Autodesk Inventor part; units mm, degrees
ref_plane "YZ Plane" through (0, 0, 0) normal (1, 0, 0) x (0, 1, 0)
ref_plane "XZ Plane" through (0, 0, 0) normal (0, 1, 0) x (-1, 0, 0)
ref_plane "XY Plane" through (0, 0, 0) normal (0, 0, 1) x (1, 0, 0)
sketch "Sketch1" plane through (0, 0, 0) normal (0, 1, 0) x (-1, 0, 0)
  line L0 (0, 0) -> (-58, 0)
  line L1 (-58, 0) -> (-58, -20)
  line L2 (-58, -20) -> (0, -20)
  line L3 (0, -20) -> (0, 0)
  line L4 (-58, -10) -> (-54, -10) construction
  arc A0 (-56, -11.8875) -> (-52, -11.8875) centre (-54, -10) ccw
  line L5 (-58, -10) -> (-56, -10) construction
  line L6 (-56, -10) -> (-56, -11.8875)
  line L7 (-56, -10) -> (-56, -8.1125)
  line L8 (-54, -10) -> (-52, -10) construction
  line L9 (-52, -10) -> (-52, -11.8875)
  line L10 (-52, -10) -> (-52, -8.1125)
  arc A1 (-52, -8.1125) -> (-56, -8.1125) centre (-54, -10) ccw
  arc A2 (-58, -12.5617) -> (-58, -7.4383) centre (-54, -10) ccw
  line L11 (0, 0) -> (-10, 0) construction
  line L12 (-10, 0) -> (-10, -5) construction
  line L13 (-10, -20) -> (-10, -15) construction
  circle A3 centre (-10, -5) radius 2.75
  circle A4 centre (-10, -15) radius 2.75
  line L14 (-54, -10) -> (-54, -11.925) construction
  line L15 (-54, -10) -> (-54, -8.075) construction
  circle A5 centre (-54, -8.075) radius 0.3
  circle A6 centre (-54, -11.925) radius 0.3
  line L16 (-58, -10) -> (-31.5, -10) construction
  line L17 (-33.5, -10) -> (-24.5, -10) construction
  line L18 (-35.5, -20) -> (-35.5, 0)
  line L19 (-24.5, -20) -> (-24.5, 0)
  line L20 (-31.5, -10) -> (-33.5, -10) construction
  line L21 (-33.5, -10) -> (-35.5, -10) construction
  line L22 (-24.5, 0) -> (-35.5, 0)
  line L23 (-35.5, 0) -> (-35.5, -20)
  line L24 (-35.5, -20) -> (-24.5, -20)
  line L25 (-24.5, -20) -> (-24.5, 0)
  dimension "d0" = 58
  dimension "d1" = 20
  dimension "d2" = 4
  dimension "d4" = 2
  dimension "d5" = 2
  dimension "d7" = 10
  dimension "d8" = 5
  dimension "d9" = 5
  dimension "d10" = 5.5
  dimension "d11" = 5.5
  dimension "d18" = 1.925
  dimension "d19" = 1.925
  dimension "d20" = 0.6
  dimension "d21" = 0.6
  dimension "d24" = 26.5
  dimension "d25" = 9
  dimension "d32" = 2
  dimension "d33" = 2
extrude "Extrusion2" add sketch "Sketch1" against normal blind 8 contours A2 L1
extrude "Extrusion3" add sketch "Sketch1" along normal blind 5 contours A2 L1
extrude "Extrusion4" add sketch "Sketch1" against normal blind 8 contours L6 L7 A1 L10 L9 A0
extrude "Extrusion8" add sketch "Sketch1" against normal blind 8 contours L3 L2 L19 L0 | L18 L2 L1 A2 L0
extrude "Extrusion9" add sketch "Sketch1" against normal blind 2.5 contours L19 L2 L18 L0
properties part number "LDR_Holder"
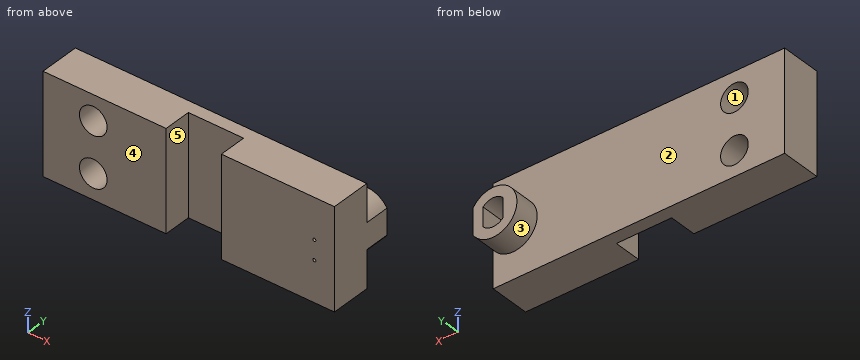
Read the model definition and answer for the solid it produces. Units are mm, in the model's axes. Face numbers are marked on the shaded views. A direction names the side the tool comes from. Give positions to 0.01 mm unless a question says otherwise; leave off trailing zeros. Write each loop counter-clockwise with the first axis right and the second up, starting at its lowest first coordinate (ties: lowest second). Pieces come first, ordered by that corner, then holes. Notation, with made-up numbers: (67, 65) - (103, 65) arc R8 cw to (103, 73) - close; hole circle Ø1 at (-18, 65.25). An arc over 180 degrees is marked (long way). Answer in a Markdown table with one row per item. Add a question column.
Item 1: Section D-D, the plane z = -18.5 is taken. Write down the section's boundary in (x, y).
Item 2: Find the intervals of material crossed by L1, parallel to Z at x = 54, y = -1.75 (3 decimals); L2, parallel to Z at x = 10, y = -6; L3, parallel to X at y = -5.25, z = -1, in increasing order.
Item 3: Flat-ended cylindrical pins translate along their axes: P1, Ø4, axis at y = 3, z = -10, coming from the -X side; P2, Ø4, axis at x = 51, z = -3, coming from the +Y side. Find the tip coordinate at first contact, or state that the pin passes through.
Item 4: Section A-A, the plane x = 10 is taken. Write down the section's boundary in (y, z), and give its area (3 significant figures).
Item 5: A tool of negligible diameter and unlimited length cuts with its end or side. For the marked faces 4 and 5, from which of +Z, -Z, +X, -X, +Y, -Y can it reach the whole face along a straight path? Write none if from no direction.
Item 6: Determine the mould class of the marked faces 1, 2 and 3 for opening direction Z: pulls with the +Z half, pulls with the -Z half, needs draft (parallel to the pull), parting line crosses it, or undercut.
Item 7: Section B-B, the plane z = -10 is taken. Write down the section's boundary in (x, y), and give its area (3 significant figures).
Item 8: Section C-C, the plane y = 2.25 is taken. Write down the section's boundary in (x, z).
Recorded:
| question | item | result |
|---|---|---|
| 1 | outline | (0, -8) - (24.5, -8) - (24.5, -2.5) - (35.5, -2.5) - (35.5, -8) - (58, -8) - (58, 0) - (0, 0) - close |
| 2 | L1 | z = -20 to -12.225, -11.625 to -8.375, -7.775 to 0 |
| 2 | L2 | z = -20 to -17.75, -12.25 to -7.75, -2.25 to 0 |
| 2 | L3 | x = 0 to 24.5, 35.5 to 58 |
| 3 | P1 | stops at x = 49.25 |
| 3 | P2 | stops at y = 0 |
| 4 | outline | (-8, -20) - (0, -20) - (0, -17.75) - (-8, -17.75) - close; (-8, -12.25) - (0, -12.25) - (0, -7.75) - (-8, -7.75) - close; (-8, -2.25) - (0, -2.25) - (0, 0) - (-8, 0) - close |
| 4 | area | 72.0 mm2 |
| 5 | face 4 | +Z, -Z, +X, -X, -Y |
| 5 | face 5 | +Z, -Z, -Y |
| 6 | face 1 | undercut |
| 6 | face 2 | needs draft |
| 6 | face 3 | parting line crosses it |
| 7 | outline | (0, -8) - (24.5, -8) - (24.5, -2.5) - (35.5, -2.5) - (35.5, -8) - (58, -8) - (58, 5) - (56, 5) - (56, 0) - (52, 0) - (52, 5) - (49.25, 5) - (49.25, 0) - (0, 0) - close |
| 7 | area | 427 mm2 |
| 8 | outline | (58, -12.56) - (58, -7.44) arc R4.75 ccw (long way) to start; hole (52, -11.89) arc R2.75 ccw to (56, -11.89) - (56, -8.11) arc R2.75 ccw to (52, -8.11) - close |
